from build123d import *

# Parameters (mm, degrees)
SKETCH1_R                = 4
BOSS_EXTRUDE1_DEPTH      = 35
BOSS_EXTRUDE2_DEPTH      = 4
BOSS_EXTRUDE2_DEPTH_BACK = 4
SKETCH4_W                = 3
SKETCH4_H                = 5.4
BOSS_EXTRUDE3_DEPTH      = 18


with BuildPart() as part:
    # Sketch1 → Boss-Extrude1 (new body)
    with BuildSketch(Plane.XY):
        Circle(SKETCH1_R)
    extrude(amount=BOSS_EXTRUDE1_DEPTH)

    # Sketch2 → Boss-Extrude2 (add, two sides)
    with BuildSketch(Plane(origin=(0, 0, 0), x_dir=(0, 0, -1), z_dir=(1, 0, 0))) as boss_extrude2_sk:
        Polygon((5.4499841, 12.71997456), (-2.5, 0), (0, 0), (6.3874841, 10.21997456), (10.4499841, 10.21997456), (10.4499841, 12.71997456), (7.9499841, 12.71997456), align=None)
    extrude(amount=BOSS_EXTRUDE2_DEPTH)
    extrude(boss_extrude2_sk.sketch, amount=-BOSS_EXTRUDE2_DEPTH_BACK)

    # Sketch4 → Boss-Extrude3 (add)
    with BuildSketch(Plane.XY.offset(35)):
        with Locations((0, 2.7)):
            Rectangle(SKETCH4_W, SKETCH4_H)
    extrude(amount=-BOSS_EXTRUDE3_DEPTH)


solid = part.part
Could you check a few things on this model? Use its own coordinates, in mm. A direction names the side the tool comes from. Coordinates: 2 decimals unless noted, no trailing zeros. Loops run counter-clockwise (first coordinate to the right, second up) from the corner with the lowest first, then second, coordinate; pieces in that order, holes last.
1. Imagine slicing it at B-B (y = 2.5). Please give me the cut outline in (x, z), and give its area (3 significant figures).
2. For faces 1 (the face through (1.5, 5, 26)), 2 (the face through (0, -2, 0)), 3 (the face through (-1.5, 5, 26)), which set-ups out of +Z, -Z, +X, -X, +Y, -Y let a thin tool reach every point of the face, with its end or its side?
3. For P1, Ø4.5, axis at x = -1, y = -2, coming from the -Z side; P2, Ø1.2, axis at x = 0.5, z = -9, coming from the -Y side; P3, Ø1.4, axis at x = 0, y = 4, coming from the -Z side, each with a flat end and sliding along its axis, tell me the tip position at first contact or that it passes through.
4. Imagine slicing it at D-D (x = 2.25). Please give me the cut outline in (y, z), and give its area (3 significant figures).
5. I need wall thicknesses on L1, parallel to Y at x = 0, z = 9.5; L2, parallel to Z at x = 2.75, y = -2.75; L3, parallel to Y at x = -1, z = 12. Which ranges of each line are inside material? Lowest first, please.
6. Imagine slicing it at C-C (z = 30.5). Please give me the cut outline in (x, y), and give its area (3 significant figures).
7. Imagine slicing it at A-A (x = 0). Please give me the cut outline in (y, z).
Computed values:
1. outline: (-4, -1.56) - (4, -1.56) - (4, 0.94) - (3.12, 0.94) - (3.12, 35) - (-3.12, 35) - (-3.12, 0.94) - (-4, 0.94) - close
1. area: 233 mm2
2. face 1: +Z, +X, +Y
2. face 2: -Z, +X, -X, -Y
2. face 3: +Z, -X, +Y
3. P1: stops at z = -0.16
3. P2: stops at y = 10.22
3. P3: stops at z = -2.94
4. outline: (-3.31, 0) - (0, 0) - (10.22, -6.39) - (10.22, -10.45) - (12.72, -10.45) - (12.72, -5.45) - (3.31, 0.43) - (3.31, 35) - (-3.31, 35) - close
4. area: 267 mm2
5. L1: y = -4 to 4
5. L2: z = 0 to 35
5. L3: y = -3.87 to 3.87
6. outline: (-1.5, 3.71) arc R4 ccw (long way) to (1.5, 3.71) - (1.5, 5.4) - (-1.5, 5.4) - close
6. area: 54.8 mm2
7. outline: (-4, 0) - (0, 0) - (10.22, -6.39) - (10.22, -10.45) - (12.72, -10.45) - (12.72, -5.45) - (4, 0) - (4, 17) - (5.4, 17) - (5.4, 35) - (-4, 35) - close
